```python
from build123d import *

# Parameters (mm, degrees)
SKETCH1_W           = 47
SKETCH1_H           = 22
SKETCH1_R           = 8
BOSS_EXTRUDE1_DEPTH = 1
BOSS_EXTRUDE2_START = 1
SKETCH1_3_R         = 8
BOSS_EXTRUDE2_DEPTH = 12
SKETCH2_3_R         = 1.5
CUT_EXTRUDE1_DEPTH  = 1
FILLET1_R           = 3.5
SKETCH3_W           = 10
SKETCH3_H           = 6
BOSS_EXTRUDE3_DEPTH = 6
SKETCH4_W           = 8
SKETCH4_H           = 5
BOSS_EXTRUDE4_DEPTH = 2.5
SKETCH5_R           = 0.75
BOSS_EXTRUDE5_DEPTH = 3


with BuildPart() as part:
    # Sketch1 → Boss-Extrude1 (new body)
    # profile 1 of 3: a face of its own
    with BuildSketch(Plane.XY):
        Rectangle(SKETCH1_W, SKETCH1_H)
        with Locations((-11, 0)):
            Circle(SKETCH1_R, mode=Mode.SUBTRACT)
        with Locations((11, 0)):
            Circle(SKETCH1_R, mode=Mode.SUBTRACT)
    # profile 2 of 3: a face of its own
    with BuildSketch(Plane.XY):
        with Locations((11, 0)):
            Circle(SKETCH1_R)
    # profile 3 of 3: a face of its own
    with BuildSketch(Plane.XY):
        with Locations((-11, 0)):
            Circle(SKETCH1_R)
    extrude(amount=BOSS_EXTRUDE1_DEPTH)

    # Sketch1<3> → Boss-Extrude2 (add)
    with BuildSketch(Plane.XY.offset(BOSS_EXTRUDE2_START)):
        with Locations((11, 0)):
            Circle(SKETCH1_3_R)
        with Locations((-11, 0)):
            Circle(SKETCH1_3_R)
    extrude(amount=BOSS_EXTRUDE2_DEPTH)

    # Sketch2<3> → Cut-Extrude1 (cut)
    with BuildSketch(Plane.XY):
        with Locations((20, 7.5)):
            Circle(SKETCH2_3_R)
        with Locations((-20, 7.5)):
            Circle(SKETCH2_3_R)
        with Locations((-20, -7.5)):
            Circle(SKETCH2_3_R)
        with Locations((20, -7.5)):
            Circle(SKETCH2_3_R)
    extrude(amount=CUT_EXTRUDE1_DEPTH, mode=Mode.SUBTRACT)

    # Fillet1
    fillet1_edges = [part.edges().sort_by_distance(p)[0] for p in [
        (-23.5, 11, 0.5),
        (23.5, 11, 0.5),
        (23.5, -11, 0.5),
        (-23.5, -11, 0.5),
    ]]
    fillet(fillet1_edges, radius=FILLET1_R)

    # Sketch3 → Boss-Extrude3 (add)
    with BuildSketch(Plane(origin=(0, 0, 0), x_dir=(-1, 0, 0), z_dir=(0, 0, -1))):
        with Locations((0, -8)):
            Rectangle(SKETCH3_W, SKETCH3_H)
    extrude(amount=BOSS_EXTRUDE3_DEPTH)

    # Sketch4 → Boss-Extrude4 (add)
    with BuildSketch(Plane(origin=(0, 0, -6), x_dir=(-1, 0, 0), z_dir=(0, 0, -1))):
        with Locations((0, -7.5)):
            Rectangle(SKETCH4_W, SKETCH4_H)
    extrude(amount=BOSS_EXTRUDE4_DEPTH)

    # Sketch5 → Boss-Extrude5 (add)
    with BuildSketch(Plane(origin=(0, 0, -8.5), x_dir=(-1, 0, 0), z_dir=(0, 0, -1))):
        with Locations((-2, -8)):
            Circle(SKETCH5_R)
        with Locations((0, -8)):
            Circle(SKETCH5_R)
        with Locations((2, -8)):
            Circle(SKETCH5_R)
    extrude(amount=BOSS_EXTRUDE5_DEPTH)


solid = part.part
```
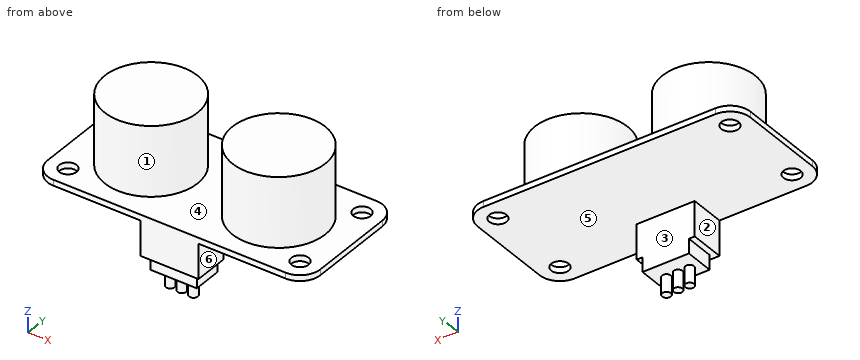
Check sheet for the modelled part. Datum: model origin and axes. Units: mm. Face numbers are marked on the shaded views. A direction names the side the tool comes from. Coordinates: 2 decimals unless noted, no trailing zeros. Loops run counter-clockwise (first coordinate to the right, second up) from the corner with the lowest first, then second, coordinate; pieces in that order, holes last.
1) Gauge pin test, flat ends, axial feed: pin 1 (5 mm diameter, centred on x = -20, y = 7.5, fed in from +Z); pin 2 (1.2 mm diameter, centred on y = -7.5, z = -8, fed in from -X); pin 3 (5 mm diameter, centred on x = -5.5, y = 3, fed in from -Z). Record the tip position at first contact, or that the pin passes through.
2) Sectioned sample at C-C (y = -4.25). Record the boundary of the cut face in (x, z), and give its area (3 significant figures).
3) Material ranges on probe 1 along Y at (x, z) = (-20, 0.5); probe 2 along Z at (x, y) = (11.5, 3.25); probe 3 along Z at (x, y) = (-2, 1), recorded low to high.
4) Sectioned sample at B-B (x = 11). Record the boundary of the cut face in (y, z), and give its area (3 significant figures).
5) Sectioned sample at A-A (z = 6.5). Record the boundary of the cut face in (x, y).
6) Release check for a two-part mould opening along X. For the marked faces 4, 5 and 6 record: released by +X, released by -X, zero draft, split by the parting line, or undercut.
7) Sectioned sample at D-D (z = -0.5). Record the boundary of the cut face in (x, y).
8) Access from +Z, -Z, +X, -X, +Y, -Y to the whole of each face (thin tool, end or side, straight path). Record for the marked faces 1, 2 and 3.
Check sheet entries:
1. pin 1: stops at z = 1
1. pin 2: stops at x = -4
1. pin 3: stops at z = 0
2. outline: (-23.5, 0) - (23.5, 0) - (23.5, 1) - (17.78, 1) - (17.78, 13) - (4.22, 13) - (4.22, 1) - (-4.22, 1) - (-4.22, 13) - (-17.78, 13) - (-17.78, 1) - (-23.5, 1) - close
2. area: 372 mm2
3. probe 1: y = -11 to -9, -6 to 6, 9 to 11
3. probe 2: z = 0 to 13
3. probe 3: z = 0 to 1
4. outline: (-11, 0) - (11, 0) - (11, 1) - (8, 1) - (8, 13) - (-8, 13) - (-8, 1) - (-11, 1) - close
4. area: 214 mm2
5. outline: circle Ø16 at (-11, 0); circle Ø16 at (11, 0)
6. face 4: undercut
6. face 5: zero draft
6. face 6: released by +X
7. outline: (-5, -11) - (5, -11) - (5, -5) - (-5, -5) - close
8. face 1: +Z
8. face 2: -Z, -X, +Y, -Y
8. face 3: -Z, +X, -X, +Y
